Source: CAD feature listing. Evaluate the final solid. Frame: model axes, mm. A direction names the side the tool comes from. Give positions to 0.01 mm unless a question says otherwise; leave off trailing zeros. Order: outer loops, then holes, each group sorted by start corner. A loop starts at its lowest first (then second) coordinate and runs counter-clockwise, first axis right, second up.
1) Section C-C, the plane y = 7. Return loops of the section in (x, z).
2) First-contact query: P1, Ø1, axis at x = 20, z = 29.5, coming from the +Y side; P2, Ø1.5, axis at y = 7, z = 4.5, coming from the -X side; P3, Ø5, axis at x = 48, y = 7.5, coming from the -Z side. Flat tips, straight axial feed; report the tip coordinate or a pass-through.
3) Access query for faces 1 (the face through (-35, -9, 19)), 2 (the face through (31, 0, 3)), 3 (the face through (84.02, 1.62, 1.48)). Directions: +Z, -Z, +X, -X, +Y, -Y. A direction counts if a zero-diameter tool reaches every point of the face in a straight line with its end or side. Return the directions, or none.
4) Section B-B, the plane z = 25. Return loops of the section in (x, y).
5) Section A-A, the plane x = 76. Return loops of the section in (y, z), plus the area to 3 significant figures.
6) Draft query along Y for faces 4 (the face through (-1, 0, 41)), 5 (the face through (-73.6, -1.8, 39.5)), 6 (the face through (-30.98, 1.62, 1.48)). Return one class per face: released by +Y, released by -Y, zero draft, split by the parting line, or undercut.
7) Section D-D, the plane x = 40.5. Return loops of the section in (y, z), plus the area to 3 significant figures.
8) Material intervals for line 1 (Y direction, x = -76, z = 39.55); line 2 (Z direction, x = 30, y = 3.25); line 3 (Z direction, x = 39.5, y = 8), sorted ascending.
```python
from build123d import *
from OCP.BRepFilletAPI import BRepFilletAPI_MakeChamfer

# Parameters (mm, degrees)
SKICA1_W                      = 190
SKICA1_H                      = 20
P_IDAT_VYSUNUT_M1_DEPTH       = 41
SKICA2_W                      = 95
SKICA2_H                      = 35
ODEBRAT_VYSUNUT_M1_DEPTH      = 17
SKICA3_W                      = 37.5
SKICA3_H                      = 20
SKICA3_W_2                    = 45
ODEBRAT_VYSUNUT_M2_DEPTH      = 38
D_RY_PRO_KOL_K_VELIKOST_MM1_D = 6
ZKOSEN_2_SIZE                 = 17
ZKOSEN_2_SIZE2                = 7.927230189
ZKOSEN_3_SIZE                 = 17
ZKOSEN_3_SIZE2                = 7.927230189


with BuildPart() as part:
    # Skica1 → Přidat vysunutím1 (new body)
    with BuildSketch(Plane.XY):
        Rectangle(SKICA1_W, SKICA1_H)
    extrude(amount=P_IDAT_VYSUNUT_M1_DEPTH)

    # Skica2 → Odebrat vysunutím1 (cut)
    with BuildSketch(Plane(origin=(0, 10, 0), x_dir=(1, 0, 0), z_dir=(0, 1, 0))):
        with Locations((-47.5, -20.5)):
            Rectangle(SKICA2_W, SKICA2_H)
        with Locations((47.5, -20.5)):
            Rectangle(SKICA2_W, SKICA2_H)
    extrude(amount=-ODEBRAT_VYSUNUT_M1_DEPTH, mode=Mode.SUBTRACT)

    # Skica3 → Odebrat vysunutím2 (cut)
    with BuildSketch(Plane(origin=(0, 0, 0), x_dir=(-1, 0, 0), z_dir=(0, 0, -1))):
        with Locations((-61.25, 0)):
            Rectangle(SKICA3_W, SKICA3_H)
        with Locations((-1.25, 0)):
            Rectangle(SKICA3_W, SKICA3_H)
        with Locations((57.5, 0)):
            Rectangle(SKICA3_W_2, SKICA3_H)
    extrude(amount=-ODEBRAT_VYSUNUT_M2_DEPTH, mode=Mode.SUBTRACT)

    # Díry pro kolík, velikost mm1 (through all)
    with Locations(Plane.XY.offset(41)):
        with Locations((-76, 0), (76, 0)):
            Hole(D_RY_PRO_KOL_K_VELIKOST_MM1_D / 2)

    # Zkosení2: one chamfer whose edges measure the first distance from different faces: ONE call of the kernel's chamfer builder (chamfer() names one face for all edges)
    zkosen_2_edges_1 = [part.edges().sort_by_distance(p)[0] for p in [
        (-35, 10, 1.5),
    ]]
    zkosen_2_side_1 = [part.faces().sort_by_distance(p)[0] for p in [
        (-35, 0, 0.429418211),
    ]]
    zkosen_2_edges_2 = [part.edges().sort_by_distance(p)[0] for p in [
        (20, 10, 1.5),
    ]]
    zkosen_2_side_2 = [part.faces().sort_by_distance(p)[0] for p in [
        (20, 0, 0.429418211),
    ]]
    zkosen_2_edges_3 = [part.edges().sort_by_distance(p)[0] for p in [
        (80, 10, 1.5),
    ]]
    zkosen_2_side_3 = [part.faces().sort_by_distance(p)[0] for p in [
        (80, 0, 0.429418211),
    ]]
    zkosen_2 = BRepFilletAPI_MakeChamfer(part.part.solid().wrapped)
    for e in zkosen_2_edges_1:
        zkosen_2.Add(ZKOSEN_2_SIZE, ZKOSEN_2_SIZE2, e.wrapped, zkosen_2_side_1[0].wrapped)  # the first distance lies on this face
    for e in zkosen_2_edges_2:
        zkosen_2.Add(ZKOSEN_2_SIZE, ZKOSEN_2_SIZE2, e.wrapped, zkosen_2_side_2[0].wrapped)  # the first distance lies on this face
    for e in zkosen_2_edges_3:
        zkosen_2.Add(ZKOSEN_2_SIZE, ZKOSEN_2_SIZE2, e.wrapped, zkosen_2_side_3[0].wrapped)  # the first distance lies on this face
    add(Compound.cast(zkosen_2.Shape()), mode=Mode.REPLACE)

    # Zkosení3: one chamfer whose edges measure the first distance from different faces: ONE call of the kernel's chamfer builder (chamfer() names one face for all edges)
    zkosen_3_edges_1 = [part.edges().sort_by_distance(p)[0] for p in [
        (-80, 10, 1.5),
    ]]
    zkosen_3_side_1 = [part.faces().sort_by_distance(p)[0] for p in [
        (-80, 0, 0.429418211),
    ]]
    zkosen_3_edges_2 = [part.edges().sort_by_distance(p)[0] for p in [
        (-17.5, 10, 1.5),
    ]]
    zkosen_3_side_2 = [part.faces().sort_by_distance(p)[0] for p in [
        (-17.5, 0, 0.429418211),
    ]]
    zkosen_3_edges_3 = [part.edges().sort_by_distance(p)[0] for p in [
        (42.5, 10, 1.5),
    ]]
    zkosen_3_side_3 = [part.faces().sort_by_distance(p)[0] for p in [
        (42.5, 0, 0.429418211),
    ]]
    zkosen_3 = BRepFilletAPI_MakeChamfer(part.part.solid().wrapped)
    for e in zkosen_3_edges_1:
        zkosen_3.Add(ZKOSEN_3_SIZE, ZKOSEN_3_SIZE2, e.wrapped, zkosen_3_side_1[0].wrapped)  # the first distance lies on this face
    for e in zkosen_3_edges_2:
        zkosen_3.Add(ZKOSEN_3_SIZE, ZKOSEN_3_SIZE2, e.wrapped, zkosen_3_side_2[0].wrapped)  # the first distance lies on this face
    for e in zkosen_3_edges_3:
        zkosen_3.Add(ZKOSEN_3_SIZE, ZKOSEN_3_SIZE2, e.wrapped, zkosen_3_side_3[0].wrapped)  # the first distance lies on this face
    add(Compound.cast(zkosen_3.Shape()), mode=Mode.REPLACE)


solid = part.part
```
From the geometry:
1. outline: (-95, 0) - (-86.53, 0) - (-86.53, 3) - (-95, 3) - close; (-95, 38) - (95, 38) - (95, 41) - (-95, 41) - close; (-28.47, 0) - (-24.03, 0) - (-24.03, 3) - (-28.47, 3) - close; (26.53, 0) - (35.97, 0) - (35.97, 3) - (26.53, 3) - close; (86.53, 0) - (95, 0) - (95, 3) - (86.53, 3) - close
2. P1: stops at y = -7
2. P2: passes through
2. P3: stops at z = 38
3. face 1: -Z, +Y, -Y
3. face 2: +X, -X, +Y
3. face 3: -Z, +Y
4. outline: (-95, -10) - (-80, -10) - (-80, -7) - (-95, -7) - close; (-35, -10) - (-17.5, -10) - (-17.5, -7) - (-35, -7) - close; (20, -10) - (42.5, -10) - (42.5, -7) - (20, -7) - close; (80, -10) - (95, -10) - (95, -7) - (80, -7) - close
5. outline: (-10, 38) - (-3, 38) - (-3, 41) - (-10, 41) - close; (3, 38) - (10, 38) - (10, 41) - (3, 41) - close
5. area: 42.0 mm2
6. face 4: zero draft
6. face 5: undercut
6. face 6: released by +Y
7. outline: (-10, 0) - (-2.71, 0) - (-2.71, 3) - (-7, 3) - (-7, 38) - (10, 38) - (10, 41) - (-10, 41) - close
7. area: 187 mm2
8. line 1: y = -10 to -3, 3 to 10
8. line 2: z = 0 to 3, 38 to 41
8. line 3: z = 38 to 41
